The listing builds one solid part. Answer for the finished solid, in the listing's coordinates (mm). Face numbers are marked on the shaded views. A direction names the side the tool comes from. Coordinates: 2 decimals unless noted, no trailing zeros. Order: outer loops, then holes, each group sorted by start corner. A loop starts at its lowest first (then second) coordinate and runs counter-clockwise, first axis right, second up. Notation, with made-up numbers: (6.25, 81.5) - (60.25, 81.5) arc R17 cw to (60.25, 86.5) - close; hole circle Ø3 at (37.25, 61). An arc over 180 degrees is marked (long way). One line per item, written item: value. Start each with the question number.
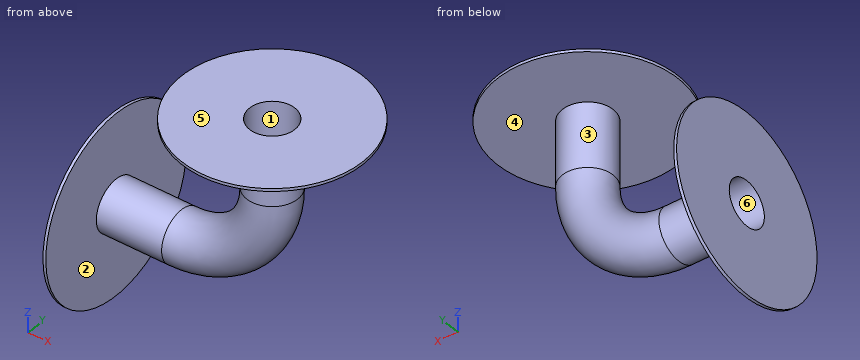
```python
from build123d import *

# Parameters (mm, degrees)
SKETCH1_R           = 14.2875
SKETCH1_R_2         = 12.7
REVOLVE1_ANGLE      = 90
SKETCH2_R           = 14.2875
SKETCH2_R_2         = 12.7
BOSS_EXTRUDE1_DEPTH = 38.1
SKETCH3_R           = 14.2875
SKETCH3_R_2         = 12.7
BOSS_EXTRUDE2_DEPTH = 38.1
BOSS_EXTRUDE3_START = -1.5875
SKETCH4_R           = 50.8
SKETCH4_R_2         = 12.7
BOSS_EXTRUDE3_DEPTH = 1.5875
BOSS_EXTRUDE4_START = -1.5875
SKETCH5_R           = 50.8
SKETCH5_R_2         = 12.7
BOSS_EXTRUDE4_DEPTH = 1.5875


with BuildPart() as part:
    # Sketch1 → Revolve1 (revolve)
    with BuildSketch(Plane(origin=(0, 0, 0), x_dir=(0, 0, -1), z_dir=(1, 0, 0))):
        Circle(SKETCH1_R)
        Circle(SKETCH1_R_2, mode=Mode.SUBTRACT)
    revolve(axis=Axis((0, 0, 50.8), (0, -1, 0)), revolution_arc=REVOLVE1_ANGLE)

    # Sketch2 → Boss-Extrude1 (add)
    with BuildSketch(Plane.XY.offset(50.8)):
        with Locations((50.8, 0)):
            Circle(SKETCH2_R)
        with Locations((50.8, 0)):
            Circle(SKETCH2_R_2, mode=Mode.SUBTRACT)
    extrude(amount=BOSS_EXTRUDE1_DEPTH)

    # Sketch3 → Boss-Extrude2 (add)
    with BuildSketch(Plane.ZY):
        with Locations(Location((0, 0, 0), (0, 0, 180))):
            Circle(SKETCH3_R)
        with Locations(Location((0, 0, 0), (0, 0, 180))):
            Circle(SKETCH3_R_2, mode=Mode.SUBTRACT)
    extrude(amount=BOSS_EXTRUDE2_DEPTH)

    # Sketch4 → Boss-Extrude3 (add)
    with BuildSketch(Plane.ZY.offset(38.1).offset(BOSS_EXTRUDE3_START)):
        Circle(SKETCH4_R)
        with Locations(Location((0, 0, 0), (0, 0, 180))):
            Circle(SKETCH4_R_2, mode=Mode.SUBTRACT)
    extrude(amount=BOSS_EXTRUDE3_DEPTH)

    # Sketch5 → Boss-Extrude4 (add)
    with BuildSketch(Plane.XY.offset(88.9).offset(BOSS_EXTRUDE4_START)):
        with Locations((50.8, 0)):
            Circle(SKETCH5_R)
        with Locations((50.8, 0)):
            Circle(SKETCH5_R_2, mode=Mode.SUBTRACT)
    extrude(amount=BOSS_EXTRUDE4_DEPTH)


solid = part.part
```
(1) Consider probe 1 along Y at (x, z) = (50.8, 63.5); probe 2 along Z at (x, y) = (12, -1); probe 3 along Z at (x, y) = (65.5, 24). Determine where each line is inside the solid, lowest interval first.
(2) The part is cut by section A-A on y = 0. Determine the outline of the cut face in (x, z) (1 decimal), plus the area to 3 significant figures.
(3) Flat-ended cylindrical pins translate along their axes: pin 1 Ø20.5 at (x, y) = (50.8, 0) entering from -Z; pin 2 Ø12 at (x, y) = (54, -37) entering from -Z; pin 3 Ø1.5 at (y, z) = (13.5, -29.5) entering from +X. Find the tip coordinate at first contact, or state that the pin passes through.
(4) For the marked faces 4, 5 and 6, determine the directions among +Z, -Z, +X, -X, +Y, -Y from which every point of the face is accessible in a straight line to the end or side of a thin tool.
(5) For a pull along Y with two mould halves and no side action, classify the marked faces 1, 2 and 3 as pulls with the +Y half, pulls with the -Y half, needs draft (parallel to the pull), parting line crosses it, or undercut.
(6) The part is cut by section B-B on z = 47. Count the separate pieces of the cut face and the enclosed holes in it, plus the area to 3 significant figures.
(7) The part is cut by section C-C on y = 39.5. Determine the outline of the cut face in (x, z), plus the area to 3 significant figures.
Completed:
1. probe 1: y = -14.29 to -12.7, 12.7 to 14.29
1. probe 2: z = -13.14 to -11.52, 14.6 to 16.28, 87.31 to 88.9
1. probe 3: z = 87.31 to 88.9
2. outline: (-38.1, -50.8) - (-36.5, -50.8) - (-36.5, -14.3) - (0, -14.3) arc R65.1 ccw to (65.1, 50.8) - (65.1, 87.3) - (101.6, 87.3) - (101.6, 88.9) - (63.5, 88.9) - (63.5, 50.8) arc R63.5 cw to (0, -12.7) - (-38.1, -12.7) - close; (-38.1, 12.7) - (0, 12.7) arc R38.1 ccw to (38.1, 50.8) - (38.1, 88.9) - (0, 88.9) - (0, 87.3) - (36.5, 87.3) - (36.5, 50.8) arc R36.5 cw to (0, 14.3) - (-36.5, 14.3) - (-36.5, 50.8) - (-38.1, 50.8) - close
2. area: 727 mm2
3. pin 1: stops at z = -0.11
3. pin 2: stops at z = 87.31
3. pin 3: stops at x = -36.51
4. face 4: none
4. face 5: +Z, +X, -X, +Y, -Y
4. face 6: -X
5. face 1: undercut
5. face 2: needs draft
5. face 3: parting line crosses it
6. separate pieces: 2
6. enclosed holes: 1
6. area: 196 mm2
7. outline: (-38.1, -31.94) - (-36.51, -31.94) - (-36.51, 31.94) - (-38.1, 31.94) - close; (18.86, 87.31) - (82.74, 87.31) - (82.74, 88.9) - (18.86, 88.9) - close
7. area: 203 mm2
